from build123d import *

# Parameters (mm, degrees)
SKETCH_1_W          = 60
SKETCH_1_H          = 30
EXTRUDE_1_DEPTH     = 10
CHAMFER_1_SIZE      = 3
SKETCH_2_R          = 3.5
CUT_EXTRUDE_1_DEPTH = 36
SKETCH_3_R          = 5.5
CUT_EXTRUDE_2_DEPTH = 6


with BuildPart() as part:
    # 草图1 → 凸台-拉伸1 (new body)
    with BuildSketch(Plane.XY):
        Rectangle(SKETCH_1_W, SKETCH_1_H)
    extrude(amount=EXTRUDE_1_DEPTH)

    # 倒角1
    chamfer_1_edges = [part.edges().sort_by_distance(p)[0] for p in [
        (-30, 0, 10),
        (0, -15, 10),
        (30, 0, 10),
        (0, 15, 10),
    ]]
    chamfer(chamfer_1_edges, length=CHAMFER_1_SIZE)

    # 草图2 → 切除-拉伸1 (cut, through all)
    with BuildSketch(Plane.XY.offset(10)):
        with Locations((-20, 0)):
            Circle(SKETCH_2_R)
        with Locations((20, 0)):
            Circle(SKETCH_2_R)
    extrude(amount=-CUT_EXTRUDE_1_DEPTH, mode=Mode.SUBTRACT)

    # 草图3 → 切除-拉伸2 (cut)
    with BuildSketch(Plane.XY.offset(10)):
        with Locations((-20, 0)):
            Circle(SKETCH_3_R)
        with Locations((20, 0)):
            Circle(SKETCH_3_R)
    extrude(amount=-CUT_EXTRUDE_2_DEPTH, mode=Mode.SUBTRACT)


solid = part.part
CAD build for the part. Positions are in the model's coordinates, mm. A direction names the side the tool comes from. Round coordinates to 2 decimals unless told otherwise and drop trailing zeros. Order: outer loops, then holes, each group sorted by start corner. A loop starts at its lowest first (then second) coordinate and runs counter-clockwise, first axis right, second up. Notation, with made-up numbers: (-24.75, 39) - (16.25, 39) arc R14 ccw to (16.25, 45) - close; hole circle Ø2 at (-17.5, -9). An arc over 180 degrees is marked (long way). Return JSON: item names as keys, results as strings.
(1) Pull direction X, two halves, no side cores. Call faces 1 (the face through (0, 0, 10)), 2 (the face through (28, 0, 9)), 3 (the face through (-14.92, -2.11, 7.04)): +X half, -X half, draft (parallel to the pull), parting line (faces both ways), or undercut.
Answer key:
{"face 1": "draft", "face 2": "+X half", "face 3": "undercut"}
(2) Wall check: probe 1 along Y at (x, z) = (20, 3.05); probe 2 along Y at (x, z) = (-20, 5.4); probe 3 along X at (y, z) = (-1.5, 4.25). Give the ranges that are in metal, low to high. Write a range as from..to.
Answer key:
{"probe 1": "y = -15..-3.5, 3.5..15", "probe 2": "y = -15..-5.5, 5.5..15", "probe 3": "x = -30..-25.29, -14.71..14.71, 25.29..30"}
(3) Pin check, flat tip, straight feed: pin 1 Ø5.5 at (x, y) = (18.5, 0.5) entering from +Z. Stop position of the tip, or through.
Answer key:
{"pin 1": "stops at z = 4"}
(4) Cut at D-D (y = 6.75). Give the cut face in (x, z).
Answer key:
{"outline": "(-30, 0) - (30, 0) - (30, 7) - (27, 10) - (-27, 10) - (-30, 7) - close"}
(5) Cut at B-B (z = 9.25). Give the cut face in (x, y), then the cut area to 3 significant figures.
Answer key:
{"outline": "(-27.75, -12.75) - (27.75, -12.75) - (27.75, 12.75) - (-27.75, 12.75) - close; hole circle Ø11 at (-20, 0); hole circle Ø11 at (20, 0)", "area": "1,230 mm^2"}
(6) Tool access for faces 4 (the face through (-16.66, 1.05, 2.03)), 5 (the face through (20, -4, 4)): list every direction of +Z, -Z, +X, -X, +Y, -Y with a clear straight run to the whole face (end or side of a thin tool).
Answer key:
{"face 4": "+Z, -Z", "face 5": "+Z"}
(7) Cut at A-A (y = 0). Give the cut face in (x, z), then the cut area to 3 significant figures.
Answer key:
{"outline": "(-30, 0) - (-23.5, 0) - (-23.5, 4) - (-25.5, 4) - (-25.5, 10) - (-27, 10) - (-30, 7) - close; (-16.5, 0) - (16.5, 0) - (16.5, 4) - (14.5, 4) - (14.5, 10) - (-14.5, 10) - (-14.5, 4) - (-16.5, 4) - close; (23.5, 0) - (30, 0) - (30, 7) - (27, 10) - (25.5, 10) - (25.5, 4) - (23.5, 4) - close", "area": "403 mm^2"}
(8) Cut at C-C (x = -20). Give the cut face in (y, z).
Answer key:
{"outline": "(-15, 0) - (-3.5, 0) - (-3.5, 4) - (-5.5, 4) - (-5.5, 10) - (-12, 10) - (-15, 7) - close; (3.5, 0) - (15, 0) - (15, 7) - (12, 10) - (5.5, 10) - (5.5, 4) - (3.5, 4) - close"}
